The figure shows three views and two pictorial views of one solid part (mm, origin at its lowest corner). Answer the questions. Coordinates: 2 decimals unless noted, no trailing zeros. Order: outer loops, then holes, each group sorted by start corner. A loop starts at its lowest first (then second) coordinate and runs counter-clockwise, first axis right, second up.
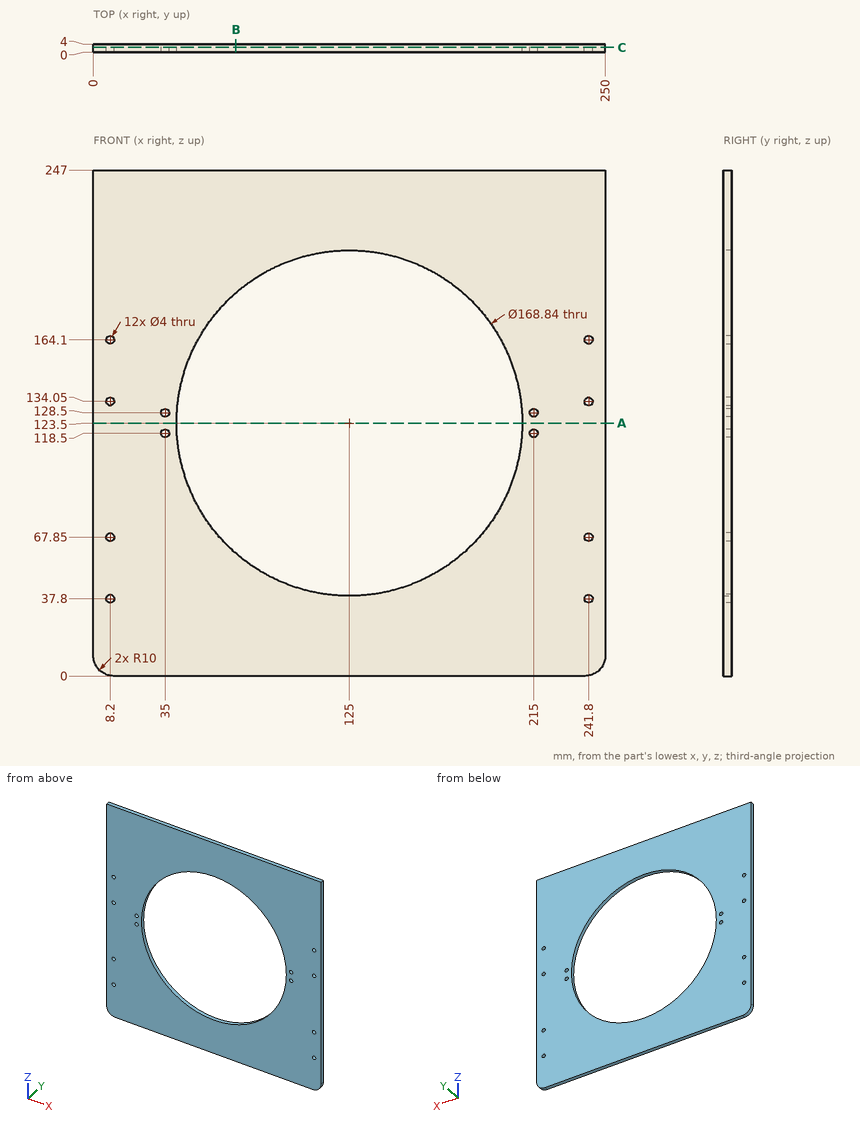
1) A cutting plane is placed at C-C, the plane y = 2.35. Count the separate pieces of the cut face and the enclosed holes in it, plus the area to 3 significant figures.
2) A cutting plane is placed at B-B, the plane x = 69.5. Write down the section's boundary in (y, z).
3) Each of these flat-tipped pins is pushed along its axis until it touches: P1, Ø5, axis at x = 8.2, z = 67.85, coming from the -Y side; P2, Ø3, axis at x = 241.8, z = 164.1, coming from the +Y side. Where does it stop, or does it pass through?
4) Straight lines are drawn through the part: probe 1 along X at (y, z) = (1.7, 37.8); probe 2 along Z at (x, y) = (215, 0.95); probe 3 along Z at (x, y) = (241.8, 1.75). For each, find the intervals that lie inside material, in ascending order.
5) A cutting plane is placed at A-A, the plane z = 123.5. Write down the section's boundary in (x, y), plus the area to 3 significant figures.
Working result:
1. separate pieces: 1
1. enclosed holes: 13
1. area: 39,200 mm2
2. outline: (0, 0) - (4, 0) - (4, 59.89) - (0, 59.89) - close; (0, 187.11) - (4, 187.11) - (4, 247) - (0, 247) - close
3. P1: stops at y = 0
3. P2: passes through
4. probe 1: x = 0 to 6.2, 10.2 to 239.8, 243.8 to 250
4. probe 2: z = 0 to 116.5, 120.5 to 126.5, 130.5 to 247
4. probe 3: z = 0.16 to 35.8, 39.8 to 65.85, 69.85 to 132.05, 136.05 to 162.1, 166.1 to 247
5. outline: (0, 0) - (40.58, 0) - (40.58, 4) - (0, 4) - close; (209.42, 0) - (250, 0) - (250, 4) - (209.42, 4) - close
5. area: 325 mm2
